```python
from build123d import *

# Parameters (mm, degrees)
F0_W     = 50
F0_H     = 50
F2_DEPTH = 22
F1_W     = 20
F1_H     = 20


# Not quite as in the source:
# - an extrude whose draft closes it to a point is written as a loft to that point


with BuildPart() as f2:
    # F0 (on Top) → F2 (new body)
    with BuildSketch(Plane.XY):
        Rectangle(F0_W, F0_H)
    extrude(amount=-F2_DEPTH)

    # F1 (on Top) → F3 section 0
    with BuildSketch(Plane.XY, mode=Mode.PRIVATE) as f3_s0:
        Rectangle(F1_W, F1_H)
    loft([f3_s0.sketch, Vertex(0, 0, -15.3986496381)], ruled=True, mode=Mode.SUBTRACT)


solid = f2.part
```
Source: CAD feature listing. Evaluate the final solid. Frame: model axes, mm. A direction names the side the tool comes from. Round coordinates to 2 decimals unless told otherwise and drop trailing zeros. Order: outer loops, then holes, each group sorted by start corner. A loop starts at its lowest first (then second) coordinate and runs counter-clockwise, first axis right, second up. Notation, with made-up numbers: (-34.5, 6) -> (20.5, 6) arc R24 ccw to (20.5, 42) -> close; hole circle Ø2 at (-11.75, 67). An arc over 180 degrees is marked (long way). One line per item, written item: value. Start each with the question number.
Q1. Section query A-A (z = -4.25). Return the cut outline in (x, y), plus the area to 3 significant figures.
Q2. Material intervals for probe 1 along X at (y, z) = (-0.5, -8); probe 2 along X at (y, z) = (6, -1.25); probe 3 along Z at (x, y) = (5.5, -8.5), sorted ascending.
Q3. Section query C-C (y = -2). Return the cut outline in (x, z), plus the area to 3 significant figures.
Q4. Section query B-B (x = -4.5). Return the cut outline in (y, z), plus the area to 3 significant figures.
Q5. Access query for faces 1 (the flat face through (0, 25, -11)), 2 (the flat face through (0.14, 6.04, -6.1)). Directions: +Z, -Z, +X, -X, +Y, -Y. A direction counts if a zero-diameter tool reaches every point of the face in a straight line with its end or side. Return the directions, or none.
Q6. Draft query along Y for faces 3 (the flat face through (6.04, -0.14, -6.1)), 4 (the flat face through (25, 0, -11)), 5 (the flat face through (0, -25, -11)). Return one class per face: pulls with the +Y half, pulls with the -Y half, needs draft (parallel to the pull), parting line crosses it, or undercut.
Q7. Pin query (flat end, axial travel): pin 1 (4 mm diameter, centred on x = 17, y = 19.5, fed in from +Z). Return the tip coordinate at first contact, or that it passes through.
Q8. Section query D-D (z = -7.5). Return the cut outline in (x, y), plus the area to 3 significant figures.
Findings below:
1. outline: (-25, -25) -> (25, -25) -> (25, 25) -> (-25, 25) -> close; hole (-7.24, -7.24) -> (7.24, -7.24) -> (7.24, 7.24) -> (-7.24, 7.24) -> close
1. area: 2,290 mm²
2. probe 1: -25 to -4.8, 4.8 to 25
2. probe 2: -25 to -9.19, 9.19 to 25
2. probe 3: -22 to -2.31
3. outline: (-25, -22) -> (25, -22) -> (25, 0) -> (10, 0) -> (2, -12.32) -> (-2, -12.32) -> (-10, 0) -> (-25, 0) -> close
3. area: 952 mm²
4. outline: (-25, -22) -> (25, -22) -> (25, 0) -> (10, 0) -> (4.5, -8.47) -> (-4.5, -8.47) -> (-10, 0) -> (-25, 0) -> close
4. area: 977 mm²
5. face 1: +Z, -Z, +X, -X, +Y
5. face 2: +Z
6. face 3: undercut
6. face 4: needs draft
6. face 5: pulls with the -Y half
7. pin 1: z = 0
8. outline: (-25, -25) -> (25, -25) -> (25, 25) -> (-25, 25) -> close; hole (-5.13, -5.13) -> (5.13, -5.13) -> (5.13, 5.13) -> (-5.13, 5.13) -> close
8. area: 2,390 mm²
